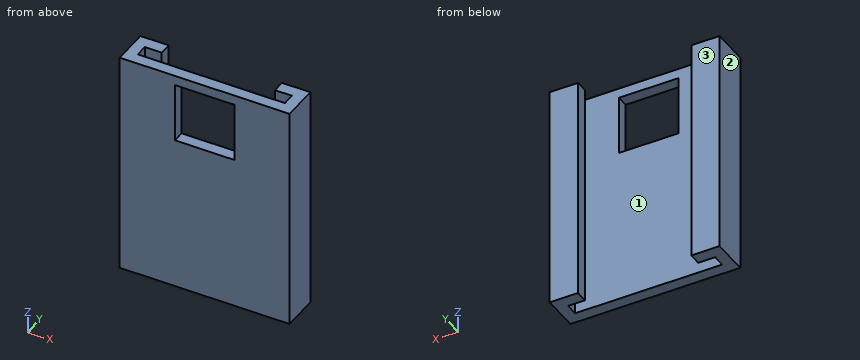
from build123d import *

# Parameters (mm, degrees)
F1_DEPTH = 50.8
F2_W     = 26.67
F2_H     = 26.67
F3_DEPTH = 16.511


with BuildPart() as f1:
    # F0 (on Top) → F1 (new body, symmetric)
    with BuildSketch(Plane.XY):
        Polygon((-38.1, 11.176), (-38.1, -5.334), (0, -5.334), (38.1, -5.334), (38.1, 11.176), (25.4, 11.176), (25.4, 5.588), (33.02, 5.588), (33.02, 0), (0, 0), (-33.02, 0), (-33.02, 5.588), (-25.4, 5.588), (-25.4, 11.176), align=None)
    extrude(amount=F1_DEPTH, both=True)

    # F2 (on face) → F3 (cut, through all)
    with BuildSketch(Plane.XZ.offset(5.334)):
        with Locations((0, 33.02)):
            Rectangle(F2_W, F2_H)
    extrude(amount=-F3_DEPTH, mode=Mode.SUBTRACT)


solid = f1.part
Here's how the part is built. I have some questions about the finished solid (model axes, mm). Face numbers are marked on the shaded views. Round coordinates to 2 decimals unless told otherwise and drop trailing zeros. Loops run counter-clockwise (first coordinate to the right, second up) from the corner with the lowest first, then second, coordinate; pieces in that order, holes last.
1. If we section it at C-C on x = 8.5: Write out the boundary of the cut face in (y, z) (3 decimals).
Answer list:
outline: (-5.334, -50.8) - (0, -50.8) - (0, 19.685) - (-5.334, 19.685) - close; (-5.334, 46.355) - (0, 46.355) - (0, 50.8) - (-5.334, 50.8) - close
2. If we section it at B-B on z = 31.5: Write out the boundary of the cut face in (x, y) (3 decimals).
Answer list:
outline: (-38.1, -5.334) - (-13.335, -5.334) - (-13.335, 0) - (-33.02, 0) - (-33.02, 5.588) - (-25.4, 5.588) - (-25.4, 11.176) - (-38.1, 11.176) - close; (13.335, -5.334) - (38.1, -5.334) - (38.1, 11.176) - (25.4, 11.176) - (25.4, 5.588) - (33.02, 5.588) - (33.02, 0) - (13.335, 0) - close
3. If I drill on line 1 along X through (y, z) = (5, 21); line 2 along Y through (x, z) = (-26, -2); line 3 along Z through (x, y) = (-7, -0.25) (3 decimals), over which ranges is the centre line in solid material (lowest first)?
Answer list:
line 1: x = -38.1 to -33.02, 33.02 to 38.1
line 2: y = -5.33 to 0, 5.59 to 11.18
line 3: z = -50.8 to 19.685, 46.355 to 50.8
4. We'd pull the mould along X, two halves only. Please class the marked faces 1, 2 and 3: +X half, -X half, draft (parallel to the pull), parting line (faces both ways), or undercut.
Answer list:
face 1: undercut
face 2: -X half
face 3: draft
5. If we section it at D-D on y = -3.5: Write out the boundary of the cut face in (x, z) (3 decimals), plus the area to 3 significant figures.
Answer list:
outline: (-38.1, -50.8) - (38.1, -50.8) - (38.1, 50.8) - (-38.1, 50.8) - close; hole (-13.335, 19.685) - (13.335, 19.685) - (13.335, 46.355) - (-13.335, 46.355) - close
area: 7,030 mm2
6. If we section it at A-A on y = 3: Write out the boundary of the cut face in (x, z).
Answer list:
outline: (-38.1, -50.8) - (-33.02, -50.8) - (-33.02, 50.8) - (-38.1, 50.8) - close; (33.02, -50.8) - (38.1, -50.8) - (38.1, 50.8) - (33.02, 50.8) - close
